from build123d import *

# Parameters (mm, degrees)
SKETCH1_W           = 50
SKETCH1_H           = 160
BOSS_EXTRUDE1_DEPTH = 47
SKETCH2_R           = 4
CUT_EXTRUDE1_DEPTH  = 10
FILLET1_R           = 3


with BuildPart() as part:
    # Sketch1 → Boss-Extrude1 (new body)
    with BuildSketch(Plane(origin=(0, 0, 0), x_dir=(1, 0, 0), z_dir=(0, 1, 0))):
        Rectangle(SKETCH1_W, SKETCH1_H)
    extrude(amount=BOSS_EXTRUDE1_DEPTH)

    # Sketch2 → Cut-Extrude1 (cut)
    with BuildSketch(Plane.XY.offset(80)):
        with Locations((-20, 31.5)):
            Circle(SKETCH2_R)
        with Locations(Location((-20, 15.5, 0), (0, 0, 180))):
            Circle(SKETCH2_R)
    extrude(amount=-CUT_EXTRUDE1_DEPTH, mode=Mode.SUBTRACT)

    # Fillet1
    fillet1_edges = [part.edges().sort_by_distance(p)[0] for p in [
        (-25, 47, 0),
        (25, 47, 0),
        (-25, 0, 0),
        (25, 0, 0),
    ]]
    fillet(fillet1_edges, radius=FILLET1_R)


solid = part.part
For this review, take the finished solid that the model builds, in its own axes (mm). A direction names the side the tool comes from. Round coordinates to 2 decimals unless told otherwise and drop trailing zeros. Write each loop counter-clockwise with the first axis right and the second up, starting at its lowest first coordinate (ties: lowest second). Pieces come first, ordered by that corner, then holes. Notation, with made-up numbers: M 56.25,66.5 L 88.25,66.5 A16 cw 88.25,94.5 Z; hole C 61.5,-14.75 d1. An arc over 180 degrees is marked long. Write item = value, one per line. Start each with the question number.
(1) We need section A-A (x = -20). Give the boundary of the cut face in (y, z), then the cut area to 3 significant figures.
(2) Clearance check with a flat-ended pin moving along its axis: pin 1 Ø9 at (x, y) = (-20.5, 14) entering from +Z. State where the tip first meets the part, or that it passes through.
(3) For line 1 along Y through (x, z) = (-20, 76.25); line 2 along X through (y, z) = (15.5, 75.75); line 3 along Z through (x, y) = (-20, 13), list the stretches that pass through material, from the lowest coordinate up.
(4) For faces 1 (the face through (0, 23, -80)), 2 (the face through (-20, 15, 70)), list the 3-axis set-ups (+Z, -Z, +X, -X, +Y, -Y) from which the entire face can be reached by the end or side of a thin tool; tool diameter is ignored.
(5) The part is to be moulded in two halves that separate along Y. For faces 3 (the face through (0, 47, -1)), 4 (the face through (-24.14, 0.9, -1.12)), 5 (the face through (-19.479, 11.534, 75.07)), say which applies: +Y half, -Y half, draft (parallel to the pull), parting line (faces both ways), or undercut.
Results found:
q1.outline = M 0,-80 L 47,-80 L 47,80 L 35.5,80 L 35.5,70 L 27.5,70 L 27.5,80 L 19.5,80 L 19.5,70 L 11.5,70 L 11.5,80 L 0,80 Z
q1.area = 7,360 mm²
q2.pin_1 = 80
q3.line_1 = 0 to 11.5, 19.5 to 27.5, 35.5 to 47
q3.line_2 = -25 to -24, -16 to 25
q3.line_3 = -80 to 70
q4.face_1 = -Z, +X, -X, +Y, -Y
q4.face_2 = +Z
q5.face_3 = +Y half
q5.face_4 = -Y half
q5.face_5 = undercut
